CAD build for the part. Positions are in the model's coordinates, mm. Face numbers are marked on the shaded views. A direction names the side the tool comes from. Round coordinates to 2 decimals unless told otherwise and drop trailing zeros. Loops run counter-clockwise (first coordinate to the right, second up) from the corner with the lowest first, then second, coordinate; pieces in that order, holes last. Notation, with made-up numbers: M -20,1 L 5,1 A32 cw 5,28 Z; hole C 22.5,35 d8. An arc over 180 degrees is marked long. Use a Markdown table: item, result. Add a question column.
(1) Which spindle directions (+Z, -Z, +X, -X, +Y, -Y) get a long thin tool onto all of the face, cutting with end or side? Do the marked faces 1 and 2. Say none if no direction does.
(2) Band-saw the part on C-C, the plane z = 15.96. Write the cut outline in (x, y), and give its area (3 significant figures).
(3) Wall check: L1, parallel to Y at x = 49, z = 5; L2, parallel to X at y = 21, z = 32; L3, parallel to X at y = 12, z = 34. Give the ranges that are in metal, low to high.
(4) Band-saw the part on B-B, the plane y = 26.5. Write the cut outline in (x, z), and give its area (3 significant figures).
(5) Band-saw the part on A-A, the plane z = 9. Write the cut outline in (x, y), and give its area (3 significant figures).
(6) Flat gauge pins, fed straight in: P1, Ø12, axis at x = -3.5, z = 12, coming from the +Y side; P2, Ø5, axis at y = 42, z = 5.5, coming from the -X side. Where does each tip first touch, or does it go through?
from build123d import *

# Parameters (mm, degrees)
SKETCH1_W                = 153
SKETCH1_H                = 37
BOSS_EXTRUDE1_DEPTH      = 49
FILLET1_R                = 5.08
SKETCH2_R                = 2.38125
BOSS_EXTRUDE2_DEPTH      = 25.4
BOSS_EXTRUDE2_DEPTH_BACK = 25.4


with BuildPart() as part:
    # Sketch1 → Boss-Extrude1 (new body)
    with BuildSketch(Plane(origin=(0, 0, 0), x_dir=(1, 0, 0), z_dir=(0, 1, 0))):
        with Locations((76.5, -18.5)):
            Rectangle(SKETCH1_W, SKETCH1_H)
    extrude(amount=BOSS_EXTRUDE1_DEPTH)

    # Fillet1
    fillet1_edges = [part.edges().sort_by_distance(p)[0] for p in [
        (153, 49, 18.5),
        (76.5, 49, 0),
        (0, 49, 18.5),
        (76.5, 0, 0),
        (153, 0, 18.5),
        (76.5, 0, 37),
        (0, 0, 18.5),
        (76.5, 49, 37),
        (0, 24.5, 0),
        (153, 24.5, 0),
        (153, 24.5, 37),
        (0, 24.5, 37),
    ]]
    fillet(fillet1_edges, radius=FILLET1_R)

    # Sketch2 → Boss-Extrude2 (add, two sides)
    with BuildSketch(Plane.ZY) as boss_extrude2_sk:
        with Locations((15.96, 43.92)):
            Circle(SKETCH2_R)
        with Locations((21.04, 43.92)):
            Circle(SKETCH2_R)
    extrude(amount=BOSS_EXTRUDE2_DEPTH)
    extrude(boss_extrude2_sk.sketch, amount=-BOSS_EXTRUDE2_DEPTH_BACK)


solid = part.part
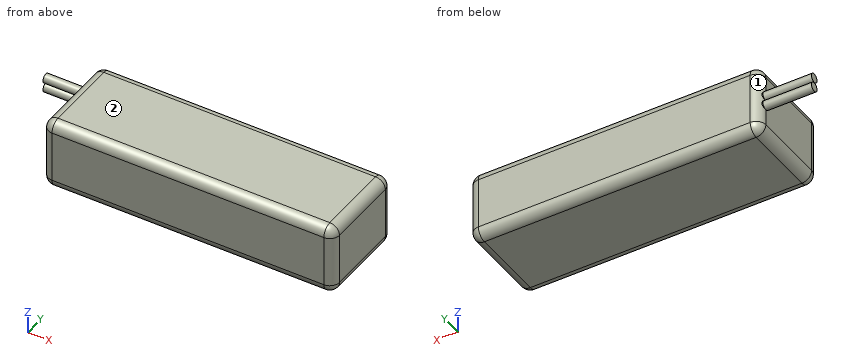
Return value:
| question | item | result |
|---|---|---|
| 1 | face 1 | -X, +Y |
| 1 | face 2 | +Z, +X, -X, +Y, -Y |
| 2 | outline | M -25.4,41.54 L 0,41.54 L 0,5.08 A5.08 ccw 5.08,0 L 147.92,0 A5.08 ccw 153,5.08 L 153,43.92 A5.08 ccw 147.92,49 L 5.08,49 A5.08 ccw 0.59,46.3 L -25.4,46.3 Z |
| 2 | area | 7,600 mm^2 |
| 3 | L1 | 0 to 49 |
| 3 | L2 | 0 to 153 |
| 3 | L3 | 0.45 to 152.55 |
| 4 | outline | M 0,5.08 A5.08 ccw 5.08,0 L 147.92,0 A5.08 ccw 153,5.08 L 153,31.92 A5.08 ccw 147.92,37 L 5.08,37 A5.08 ccw 0,31.92 Z |
| 4 | area | 5,640 mm^2 |
| 5 | outline | M 0,5.08 A5.08 ccw 5.08,0 L 147.92,0 A5.08 ccw 153,5.08 L 153,43.92 A5.08 ccw 147.92,49 L 5.08,49 A5.08 ccw 0,43.92 Z |
| 5 | area | 7,470 mm^2 |
| 6 | P1 | y = 48.3 |
| 6 | P2 | x = 0 |
